Autodesk Inventor part; units mm, degrees
ref_plane "YZ Plane" through (0, 0, 0) normal (1, 0, 0) x (0, 1, 0)
ref_plane "XZ Plane" through (0, 0, 0) normal (0, 1, 0) x (-1, 0, 0)
ref_plane "XY Plane" through (0, 0, 0) normal (0, 0, 1) x (1, 0, 0)
sketch "Sketch1" plane through (0, 0, 0) normal (0, 0, 1) x (1, 0, 0)
  line L0 (-25.9313, 51.336) -> (29.0687, 51.336)
  line L1 (29.0687, 51.336) -> (29.0687, -38.664)
  line L2 (29.0687, -38.664) -> (-25.9313, -38.664)
  line L3 (-25.9313, -38.664) -> (-25.9313, 51.336)
  circle A0 centre (-4.4697, 44.536) radius 2
  circle A1 centre (-18.7076, 12.736) radius 2
  circle A2 centre (-9.9812, 12.736) radius 2
  circle A3 centre (-4.4697, -18.464) radius 2
  line L4 (1.5687, -29.464) -> (-8.4313, -29.464)
  line L5 (-8.4313, -29.464) -> (-8.4313, -38.664)
  circle A4 centre (7.6071, 44.536) radius 2
  circle A5 centre (21.8451, 12.736) radius 2
  circle A6 centre (13.1186, 12.736) radius 2
  circle A7 centre (7.6071, -18.464) radius 2
  line L6 (1.5687, -29.464) -> (11.5687, -29.464)
  line L7 (11.5687, -29.464) -> (11.5687, -38.664)
  circle A8 centre (21.5687, 41.336) radius 1.5
  circle A9 centre (-18.4313, 41.336) radius 1.5
  circle A10 centre (21.5687, -28.664) radius 1.5
  circle A11 centre (-18.4313, -28.664) radius 1.5
  point P0 (0, 0)
  point P1 (3.1375, 0)
  dimension "d0" = 55
  dimension "d1" = 90
  dimension "d2" = 4
  dimension "d3" = 6.8
  dimension "d4" = 4
  dimension "d5" = 4
  dimension "d6" = 38.6
  dimension "d7" = 38.6
  dimension "d8" = 4
  dimension "d9" = 69.8
  dimension "d10" = 10
  dimension "d11" = 80.8
  dimension "d18" = 3
  dimension "d19" = 7.5
  dimension "d20" = 10
  dimension "d21" = 3
  dimension "d22" = 10
  dimension "d23" = 7.5
  dimension "d24" = 3
  dimension "d25" = 7.5
  dimension "d26" = 10
  dimension "d27" = 3
  dimension "d28" = 7.5
  dimension "d29" = 10
extrude "Extrusion1" add sketch "Sketch1" along normal blind 2 contours L0 L1 L2 L7 L6 L4 L5 L3 | A8 | A9 | A10 | A11
extrude "Extrusion2" add sketch "Sketch1" along normal blind 15 contours A0 | A1 | A2 | A3 | A4 | A5 | A6 | A7
extrude "Extrusion3" add sketch "Sketch1" along normal blind 7 contours L5 L4 L6 L7 L2
extrude "Extrusion4" add sketch "Sketch1" against normal blind 10 contours A8
extrude "Extrusion5" add sketch "Sketch1" against normal blind 10 contours A9
extrude "Extrusion6" add sketch "Sketch1" against normal blind 10 contours A10 | A11
properties part number "line sensor"
The model under review builds one solid part; all positions refer to its coordinate system, in mm. A direction names the side the tool comes from. Round coordinates to 2 decimals unless told otherwise and drop trailing zeros. Order: outer loops, then holes, each group sorted by start corner. A loop starts at its lowest first (then second) coordinate and runs counter-clockwise, first axis right, second up. Notation, with made-up numbers: M -15.75,86.5 L 16.25,86.5 A16 ccw 16.25,93.5 Z; hole C 61,11 d4. An arc over 180 degrees is marked long. Use a Markdown table: item, result.
1) Consider section D-D (x = 13). Write out the cut boundary in (y, z), then the cut area to 3 significant figures.
Report:
| item | result |
|---|---|
| outline | M -38.66,0 L 51.34,0 L 51.34,2 L 14.73,2 L 14.73,15 L 10.74,15 L 10.74,2 L -38.66,2 Z |
| area | 232 mm^2 |
2) Tool access review of faces 1 (the face through (2, -29.464, 4)), 2 (the face through (20.258, 13.953, 8.409)), 3 (the face through (-8.431, -34, 4)), 4 (the face through (20.07, 41.4, -4.93)): name each direction out of +Z, -Z, +X, -X, +Y, -Y from which nothing blocks a thin tool from reaching the whole face with its end or side.
Report:
| item | result |
|---|---|
| face 1 | +Z, +X, -X |
| face 2 | +Z |
| face 3 | +Z, -X, -Y |
| face 4 | -Z |
3) Draft analysis for pull direction X (two halves, no side actions). For faces 5 (the face through (-3.55, 46.31, 8.41)), 6 (the face through (-18, 41, -10)), 7 (the face through (11.569, -34, 4)), state which applies: released by +X, released by -X, zero draft, split by the parting line, or undercut.
Report:
| item | result |
|---|---|
| face 5 | undercut |
| face 6 | zero draft |
| face 7 | released by +X |
4) Consider section C-C (z = -4.75). Write out the cut boundary in (x, y), then the cut area to 3 significant figures.
Report:
| item | result |
|---|---|
| outline | C -18.43,-28.66 d3; C -18.43,41.34 d3; C 21.57,-28.66 d3; C 21.57,41.34 d3 |
| area | 28.3 mm^2 |
5) Consider section A-A (x = 0.5). Write out the cut boundary in (y, z), then the cut area to 3 significant figures.
Report:
| item | result |
|---|---|
| outline | M -38.66,0 L 51.34,0 L 51.34,2 L -29.46,2 L -29.46,7 L -38.66,7 Z |
| area | 226 mm^2 |
6) Wall thickness on line 1 along Y through (x, z) = (-4.5, 2.75); line 2 along Z through (x, y) = (2, 20); line 3 along X through (y, z) = (-35, 5.75): over which ranges is each line inside the solid? List them lowest first. Write a range as [from, to].
Report:
| item | result |
|---|---|
| line 1 | [-38.66, -29.46], [-20.46, -16.46], [42.54, 46.54] |
| line 2 | [0, 2] |
| line 3 | [-8.43, 11.57] |
7) Consider section B-B (y = 21). Write out the cut boundary in (x, z), then the cut area to 3 significant figures.
Report:
| item | result |
|---|---|
| outline | M -25.93,0 L 29.07,0 L 29.07,2 L -25.93,2 Z |
| area | 110 mm^2 |
8) Insertion check: pin 1 (8 mm diameter, centred on x = -6.5, y = 15.5, fed in from -Z); pin 2 (1.5 mm diameter, centred on y = -33, z = 4, fed in from +X); pin 3 (5 mm diameter, centred on x = -6.5, z = 9, fed in from +Y). Each pin has a flat end and moves straight along its axis. Give the tip position at first contact, or say it passes through.
Report:
| item | result |
|---|---|
| pin 1 | z = 0 |
| pin 2 | x = 11.57 |
| pin 3 | y = 46.54 |
